Could you check a few things on this drawing? It's one solid part, dimensions in mm from its lowest x, y, z. A direction names the side the tool comes from. Give positions to 0.01 mm unless a question says otherwise; leave off trailing zeros. Loops run counter-clockwise (first coordinate to the right, second up) from the corner with the lowest first, then second, coordinate; pieces in that order, holes last. Notation, with made-up numbers: M 54,80.5 L 58,80.5 A23 ccw 58,92.5 Z; hole C 77.5,40 d1. An arc over 180 degrees is marked long. Return JSON: item names as keys, results as strings. Group by question number.
1. If we section it at A-A (z = 9.9): Write out the boundary of the cut face in (x, y), plus the area to 3 significant figures.
2. If we section it at D-D (z = 2.5): Write out the boundary of the cut face in (x, y), plus the area to 3 significant figures.
3. If we mould it in two halves opening along X, with no side actions, what happens to the marked faces 3, 4 and 5? For each: +X half, -X half, draft (parallel to the pull), parting line (faces both ways), or undercut.
4. If we section it at C-C (y = 15.5): Write out the boundary of the cut face in (x, z), plus the area to 3 significant figures.
5. For pin 1 (1 mm diameter, centred on x = 8.5, z = 9.5, fed in from +Y); pin 2 (1 mm diameter, centred on x = 15, z = 12.5, fed in from +Y); pin 3 (1.5 mm diameter, centred on x = 9.5, y = 10, fed in from -Z), each with a flat end and sliding along its axis, tell me the tip position at first contact or that it passes through.
6. If we section it at B-B (x = 9.9): Write out the boundary of the cut face in (y, z), plus the area to 3 significant figures.
7. For the marked faces 1 and 2, which set-ups out of +Z, -Z, +X, -X, +Y, -Y let a thin tool reach every point of the face, with its end or its side?
8. Please list where these lines run through material, in increasing order: line 1 (Z direction, x = 10, y = 34.5); line 2 (Y direction, x = 2.75, z = 6).
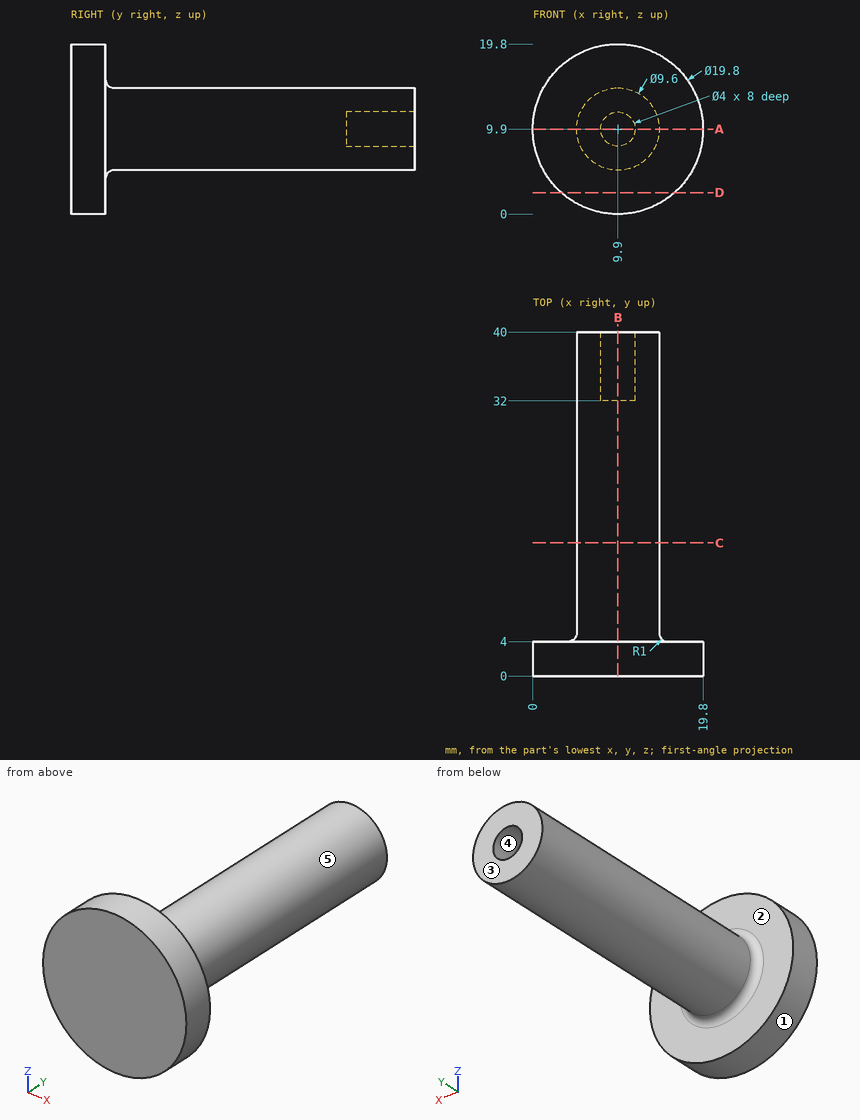
Answer:
{
 "1": {"outline": "M 0,0 L 19.8,0 L 19.8,4 L 15.7,4 A1 cw 14.7,5 L 14.7,40 L 11.9,40 L 11.9,32 L 7.9,32 L 7.9,40 L 5.1,40 L 5.1,5 A1 cw 4.1,4 L 0,4 Z", "area": "393 mm²"},
 "2": {"outline": "M 3.32,0 L 16.48,0 L 16.48,4 L 3.32,4 Z", "area": "52.6 mm²"},
 "3": {"face 3": "draft", "face 4": "undercut", "face 5": "parting line"},
 "4": {"outline": "C 9.9,9.9 d9.6", "area": "72.4 mm²"},
 "5": {"pin 1": "stops at y = 32", "pin 2": "stops at y = 4.18", "pin 3": "stops at z = 5.1"},
 "6": {"outline": "M 0,0 L 4,0 L 4,4.1 A1 cw 5,5.1 L 40,5.1 L 40,7.9 L 32,7.9 L 32,11.9 L 40,11.9 L 40,14.7 L 5,14.7 A1 cw 4,15.7 L 4,19.8 L 0,19.8 Z", "area": "393 mm²"},
 "7": {"face 1": "+Y, -Y", "face 2": "+Y"},
 "8": {"line 1": "z = 5.1 to 7.9, 11.9 to 14.7", "line 2": "y = 0 to 4"}
}
